Source: three-view drawing plus pictorial views. Frame: mm from the lowest corner of the part. Give positions to 0.01 mm unless a question says otherwise; leave off trailing zeros. Loops run counter-clockwise (first coordinate to the right, second up) from the corner with the lowest first, then second, coordinate; pieces in that order, holes last.
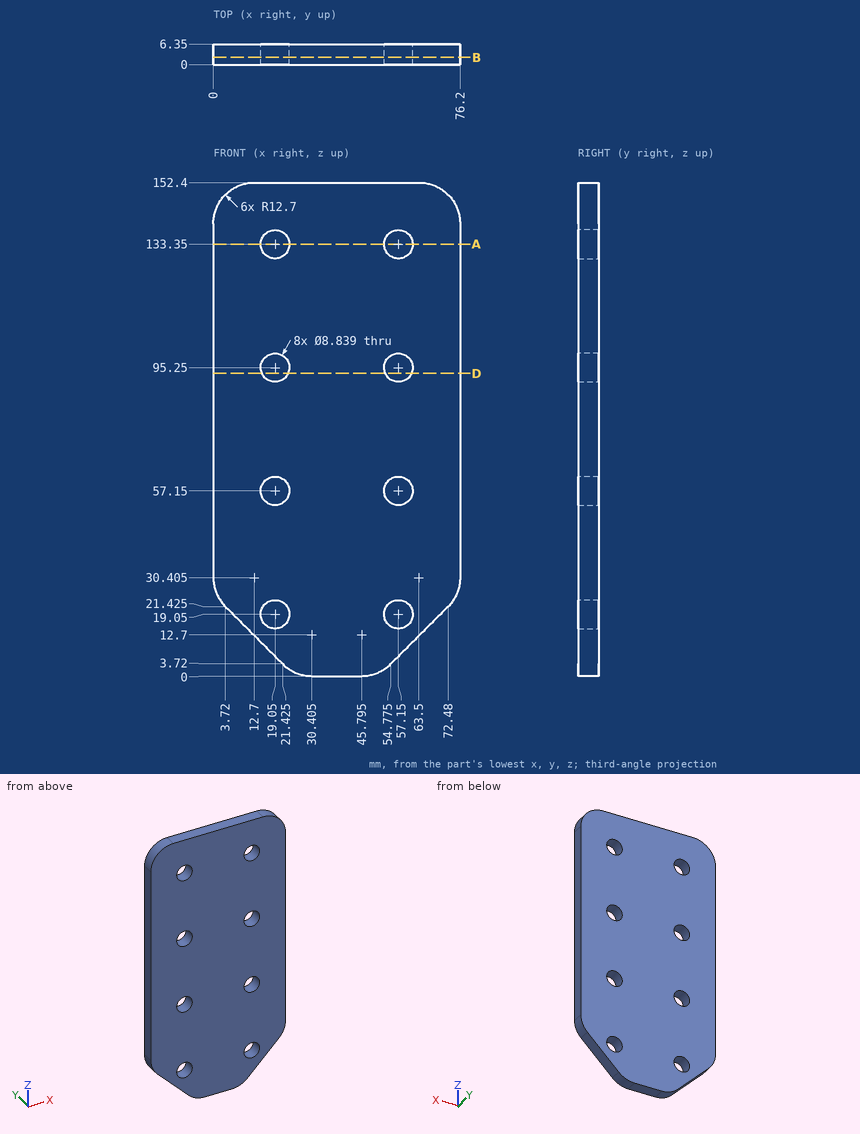
(1) Cut plane A-A (z = 133.35). Return the cut outline in (x, y).
Values follow:
outline: (0, 0) - (14.63, 0) - (14.63, 6.35) - (0, 6.35) - close; (23.47, 0) - (52.73, 0) - (52.73, 6.35) - (23.47, 6.35) - close; (61.57, 0) - (76.2, 0) - (76.2, 6.35) - (61.57, 6.35) - close
(2) Cut plane D-D (z = 93.5). Return the cut outline in (x, y), and give its area (3 significant figures).
Values follow:
outline: (0, 0) - (14.99, 0) - (14.99, 6.35) - (0, 6.35) - close; (23.11, 0) - (53.09, 0) - (53.09, 6.35) - (23.11, 6.35) - close; (61.21, 0) - (76.2, 0) - (76.2, 6.35) - (61.21, 6.35) - close
area: 381 mm2
(3) Cut plane B-B (y = 2.25). Count the separate pieces of the cut face and the enclosed holes in it, and give its area (3 significant figures).
Values follow:
separate pieces: 1
enclosed holes: 8
area: 10,400 mm2
(4) Pin query (flat end, axial travel): pin 1 Ø8 at (x, z) = (57.15, 95.25) entering from -Y; pin 2 Ø3 at (x, y) = (12.5, 1) entering from -Z (1 decimal); pin 3 Ø1 at (y, z) = (2.5, 23) entering from +X; pin 4 Ø3 at (x, y) = (13, 3) entering from -Z (1 decimal). Return the tip coordinate at first contact, or that it passes through.
Values follow:
pin 1: passes through
pin 2: stops at z = 11.1
pin 3: stops at x = 74.16
pin 4: stops at z = 10.6
(5) Ray query, probe 1 along X at (y, z) = (2.25, 57.15); probe 2 along Z at (x, y) = (15, 3.25) (1 decimal); probe 3 along Z at (x, y) = (16.5, 1.5) (1 decimal). Return the intervals inside material, ascending.
Values follow:
probe 1: x = 0 to 14.63, 23.47 to 52.73, 61.57 to 76.2
probe 2: z = 10.1 to 17.3, 20.8 to 55.4, 58.9 to 93.5, 97 to 131.6, 135.1 to 152.4
probe 3: z = 8.6 to 15.4, 22.7 to 53.5, 60.8 to 91.6, 98.9 to 129.7, 137 to 152.4
